```python
from build123d import *

# Parameters (mm, degrees)
BOSS_EXTRUDE1_DEPTH           = 1
SKETCH4_R                     = 2.3
BOSS_EXTRUDE2_DEPTH           = 2
M2_CLEARANCE_HOLE1_AT_2_COUNT = 2
M2_CLEARANCE_HOLE1_AT_2_PITCH = 12.5
M2_CLEARANCE_HOLE1_AT_3_COUNT = 2
M2_CLEARANCE_HOLE1_AT_3_PITCH = 24.43869882
M2_CLEARANCE_HOLE1_AT_4_COUNT = 2
M2_CLEARANCE_HOLE1_AT_4_PITCH = 21
BOSS_EXTRUDE3_START           = -1
BOSS_EXTRUDE3_DEPTH           = 0.75
CHAMFER1_SIZE                 = 0.4
CHAMFER1_SIZE_2               = 2
CUT_EXTRUDE2_DEPTH            = 0.8


with BuildPart() as part:
    # Sketch1 → Boss-Extrude1 (new body)
    with BuildSketch(Plane.XY):
        with BuildLine():
            Line((10.5, 12), (-10.5, 12))
            ThreePointArc((-10.5, 12), (-12.621320344, 11.121320344), (-13.5, 9))
            Line((-13.5, 9), (-13.5, -9))
            ThreePointArc((-13.5, -9), (-12.621320344, -11.121320344), (-10.5, -12))
            Line((-10.5, -12), (10.5, -12))
            ThreePointArc((10.5, -12), (12.621320344, -11.121320344), (13.5, -9))
            Line((13.5, -9), (13.5, 9))
            ThreePointArc((13.5, 9), (12.621320344, 11.121320344), (10.5, 12))
        make_face()
    extrude(amount=BOSS_EXTRUDE1_DEPTH)

    # Sketch4 → Boss-Extrude2 (add)
    with BuildSketch(Plane(origin=(0, 0, 0), x_dir=(-1, 0, 0), z_dir=(0, 0, -1))):
        with Locations((-10.5, 3.5)):
            Circle(SKETCH4_R)
        with Locations((10.5, 3.5)):
            Circle(SKETCH4_R)
        with Locations((10.5, -9)):
            Circle(SKETCH4_R)
        with Locations((-10.5, -9)):
            Circle(SKETCH4_R)
    extrude(amount=BOSS_EXTRUDE2_DEPTH)

    # Sketch3 → M2 Clearance Hole1 (revolve, cut)
    with BuildSketch(Plane(origin=(10.5, 3.5, 1), x_dir=(0, -1, 0), z_dir=(1, 0, 0))):
        Polygon((0, 0), (0, 3), (1.1, 3), (1.1, 0.965685425), (1.5, 0), align=None)
    m2_clearance_hole1 = revolve(axis=Axis((10.5, 3.5, 7.35), (0, 0, -1)), mode=Mode.SUBTRACT)

    # M2 Clearance Hole1 at 2: M2 Clearance Hole1 ×2
    with Locations(*[(0, -i * M2_CLEARANCE_HOLE1_AT_2_PITCH, 0) for i in range(1, M2_CLEARANCE_HOLE1_AT_2_COUNT)]):
        add(m2_clearance_hole1, mode=Mode.SUBTRACT)

    # M2 Clearance Hole1 at 3: M2 Clearance Hole1 ×2
    with Locations(*[Vector(-0.8592928844097065, -0.5114838597676831, 0) * (i * M2_CLEARANCE_HOLE1_AT_3_PITCH) for i in range(1, M2_CLEARANCE_HOLE1_AT_3_COUNT)]):
        add(m2_clearance_hole1, mode=Mode.SUBTRACT)

    # M2 Clearance Hole1 at 4: M2 Clearance Hole1 ×2
    with Locations(*[(-i * M2_CLEARANCE_HOLE1_AT_4_PITCH, 0, 0) for i in range(1, M2_CLEARANCE_HOLE1_AT_4_COUNT)]):
        add(m2_clearance_hole1, mode=Mode.SUBTRACT)

    # Sketch6 → Boss-Extrude3 (add)
    with BuildSketch(Plane.XY.offset(1).offset(BOSS_EXTRUDE3_START)):
        with BuildLine():
            Line((10.124367201, 2.4), (10.875632799, 2.4))
            ThreePointArc((10.875632799, 2.4), (10.5, 2.57), (10.124367201, 2.4))
        make_face()
        with BuildLine():
            Line((10.124367201, 4.6), (10.875632799, 4.6))
            ThreePointArc((10.875632799, 4.6), (10.5, 4.43), (10.124367201, 4.6))
        make_face()
        with BuildLine():
            Line((-10.124367201, 2.4), (-10.875632799, 2.4))
            ThreePointArc((-10.875632799, 2.4), (-10.5, 2.57), (-10.124367201, 2.4))
        make_face()
        with BuildLine():
            Line((-10.124367201, 4.6), (-10.875632799, 4.6))
            ThreePointArc((-10.875632799, 4.6), (-10.5, 4.43), (-10.124367201, 4.6))
        make_face()
        with BuildLine():
            Line((10.124367201, -10.1), (10.875632799, -10.1))
            ThreePointArc((10.875632799, -10.1), (10.5, -9.93), (10.124367201, -10.1))
        make_face()
        with BuildLine():
            Line((10.124367201, -7.9), (10.875632799, -7.9))
            ThreePointArc((10.875632799, -7.9), (10.5, -8.07), (10.124367201, -7.9))
        make_face()
        with BuildLine():
            Line((-10.124367201, -10.1), (-10.875632799, -10.1))
            ThreePointArc((-10.875632799, -10.1), (-10.5, -9.93), (-10.124367201, -10.1))
        make_face()
        with BuildLine():
            Line((-10.124367201, -7.9), (-10.875632799, -7.9))
            ThreePointArc((-10.875632799, -7.9), (-10.5, -8.07), (-10.124367201, -7.9))
        make_face()
    extrude(amount=-BOSS_EXTRUDE3_DEPTH)

    # Chamfer1
    # the kernel refuses this chamfer: 2, 0.4 mm, written as the material it takes off along each edge
    with BuildSketch(Plane(origin=(10.5, 3.5, -2), x_dir=(-1, 0, 0), z_dir=(0, -1, 0))) as chamfer1_piece_1_section:
        Polygon((2.3 - CHAMFER1_SIZE, 0), (2.3, -CHAMFER1_SIZE_2), (2.3, 0), align=None)
    chamfer1_piece_1 = revolve(axis=Axis((10.5, 3.5, -2), (0, 0, -1)), mode=Mode.PRIVATE)
    chamfer1_piece_1 = split(chamfer1_piece_1, bisect_by=Plane(origin=(12.610878193, 3.5, 0), z_dir=(0, 0, -1)), keep=Keep.TOP, mode=Mode.PRIVATE)
    add(chamfer1_piece_1, mode=Mode.SUBTRACT)
    with BuildSketch(Plane(origin=(-10.5, 3.5, -2), x_dir=(-1, 0, 0), z_dir=(0, -1, 0))) as chamfer1_piece_2_section:
        Polygon((2.3 - CHAMFER1_SIZE, 0), (2.3, -CHAMFER1_SIZE_2), (2.3, 0), align=None)
    chamfer1_piece_2 = revolve(axis=Axis((-10.5, 3.5, -2), (0, 0, -1)), mode=Mode.PRIVATE)
    chamfer1_piece_2 = split(chamfer1_piece_2, bisect_by=Plane(origin=(-8.389121807, 3.5, 0), z_dir=(0, 0, -1)), keep=Keep.TOP, mode=Mode.PRIVATE)
    add(chamfer1_piece_2, mode=Mode.SUBTRACT)
    with BuildSketch(Plane(origin=(-10.5, -9, -2), x_dir=(-1, 0, 0), z_dir=(0, -1, 0))) as chamfer1_piece_3_section:
        Polygon((2.3 - CHAMFER1_SIZE, 0), (2.3, -CHAMFER1_SIZE_2), (2.3, 0), align=None)
    chamfer1_piece_3 = revolve(axis=Axis((-10.5, -9, -2), (0, 0, -1)), mode=Mode.PRIVATE)
    chamfer1_piece_3 = split(chamfer1_piece_3, bisect_by=Plane(origin=(-8.389121807, -9, 0), z_dir=(0, 0, -1)), keep=Keep.TOP, mode=Mode.PRIVATE)
    add(chamfer1_piece_3, mode=Mode.SUBTRACT)
    with BuildSketch(Plane(origin=(10.5, -9, -2), x_dir=(-1, 0, 0), z_dir=(0, -1, 0))) as chamfer1_piece_4_section:
        Polygon((2.3 - CHAMFER1_SIZE, 0), (2.3, -CHAMFER1_SIZE_2), (2.3, 0), align=None)
    chamfer1_piece_4 = revolve(axis=Axis((10.5, -9, -2), (0, 0, -1)), mode=Mode.PRIVATE)
    chamfer1_piece_4 = split(chamfer1_piece_4, bisect_by=Plane(origin=(12.610878193, -9, 0), z_dir=(0, 0, -1)), keep=Keep.TOP, mode=Mode.PRIVATE)
    add(chamfer1_piece_4, mode=Mode.SUBTRACT)

    # Sketch5 → Cut-Extrude2 (cut)
    with BuildSketch(Plane(origin=(0, 0, -2), x_dir=(-1, 0, 0), z_dir=(0, 0, -1))):
        with BuildLine():
            Line((8.712564289, 4.947436899), (10.5, 3.5))
            Line((10.5, 3.5), (9.180774196, 1.615950298))
            ThreePointArc((9.180774196, 1.615950298), (8.222383442, 3.179901868), (8.712564289, 4.947436899))
        make_face()
        with BuildLine():
            Line((10.419731158, -11.298598902), (10.5, -9))
            Line((10.5, -9), (8.258948851, -9.517387425))
            ThreePointArc((8.258948851, -9.517387425), (9.037020093, -10.774736542), (10.419731158, -11.298598902))
        make_face()
        with BuildLine():
            Line((-12.674692724, 2.751193245), (-10.5, 3.5))
            Line((-10.5, 3.5), (-10.740415466, 1.212599641))
            ThreePointArc((-10.740415466, 1.212599641), (-11.931783664, 1.700001239), (-12.674692724, 2.751193245))
        make_face()
        with BuildLine():
            Line((-10.5, -6.7), (-10.5, -9))
            Line((-10.5, -9), (-8.200350301, -8.959859465))
            ThreePointArc((-8.200350301, -8.959859465), (-8.887908692, -7.359523967), (-10.5, -6.7))
        make_face()
    extrude(amount=-CUT_EXTRUDE2_DEPTH, mode=Mode.SUBTRACT)


solid = part.part
```
Could you check a few things on this model? Use its own coordinates, in mm. A direction names the side the tool comes from. Round coordinates to 2 decimals unless told otherwise and drop trailing zeros. Loops run counter-clockwise (first coordinate to the right, second up) from the corner with the lowest first, then second, coordinate; pieces in that order, holes last. Notation, with made-up numbers: (87, -25.5) - (127, -25.5) arc R23 cw to (127, -12.5) - close; hole circle Ø7 at (62, 1.5). An arc over 180 degrees is marked (long way). Answer in a Markdown table with one row per item. Add a question column.
(1) If we section it at A-A (z = 0.65): Please give me the cut outline in (x, y).
(2) I need wall thicknesses on line 1 along Y through (x, z) = (-10.5, -0.8); line 2 along Y through (x, z) = (10.5, -0.7); line 3 along X through (y, z) = (3.5, -1.15). Which ranges of each line are inside material? Lowest first, please.
(3) If we section it at B-B (y = 8.5): Please give me the cut outline in (x, z).
(4) If we mould it in two halves opening along X, with no side actions, what happens to faces 3 (the face through (12.1, -10.3, -1.2)), 4 (the face through (-12.64, -11.1, 0.49)), 5 (the face through (-12, -9, -2)), 6 (the face through (-11.43, 2.91, -0.97))? For each: pulls with the +X half, pulls with the -X half, needs draft (parallel to the pull), parting line crosses it, or undercut.
(5) If we section it at D-D (x = 9.75): State how many separate pieces and enclosed holes the cut face has, plus the area to 3 significant figures.
(6) For faces 1 (the face through (0, 0, 0)), 2 (the face through (12.6, -11.14, 0.49)), which set-ups out of +Z, -Z, +X, -X, +Y, -Y let a thin tool reach every point of the face, with its end or its side?
(7) I'm going to push a flat-ended pin straight in: pin 1 (0.9 mm diameter, centred on y = -7.5, z = -1.5, fed in from -X). Where does the tip first touch, or does it pass through?
(8) If we section it at C-C (x = -1.5): Please give me the cut outline in (y, z), plus the area to 3 significant figures.
Model answer:
| question | item | result |
|---|---|---|
| 1 | outline | (-13.5, -9) arc R3 ccw to (-10.5, -12) - (10.5, -12) arc R3 ccw to (13.5, -9) - (13.5, 9) arc R3 ccw to (10.5, 12) - (-10.5, 12) arc R3 ccw to (-13.5, 9) - close; hole circle Ø2.71 at (-10.5, -9); hole circle Ø2.71 at (-10.5, 3.5); hole circle Ø2.71 at (10.5, -9); hole circle Ø2.71 at (10.5, 3.5) |
| 2 | line 1 | y = -11.14 to -10.1, -7.9 to -6.86, 1.36 to 2.4, 4.6 to 5.64 |
| 2 | line 2 | y = -11.16 to -9.93, -8.07 to -6.84, 1.34 to 2.57, 4.43 to 5.66 |
| 2 | line 3 | x = -12.57 to -11.6, -9.4 to -8.43, 8.43 to 9.4, 11.6 to 12.57 |
| 3 | outline | (-13.5, 0) - (13.5, 0) - (13.5, 1) - (-13.5, 1) - close |
| 4 | face 3 | undercut |
| 4 | face 4 | pulls with the -X half |
| 4 | face 5 | needs draft |
| 4 | face 6 | undercut |
| 5 | separate pieces | 3 |
| 5 | enclosed holes | 0 |
| 5 | area | 28.2 mm² |
| 6 | face 1 | -Z |
| 6 | face 2 | +Z, -Z, +X, -Y |
| 7 | pin 1 | stops at x = -12.22 |
| 8 | outline | (-12, 0) - (12, 0) - (12, 1) - (-12, 1) - close |
| 8 | area | 24.0 mm² |
